from build123d import *

# Parameters (mm, degrees)
F1_DEPTH = 2057.4
F2_W     = 1651
F2_H     = 558.8
F3_DEPTH = 152.4
F4_R     = 101.6


with BuildPart() as f1:
    # F0 (on Right) → F1 (new body)
    with BuildSketch(Plane.YZ):
        Polygon((0, 939.8), (0, 0), (889, 0), (889, 558.8), (330.2, 558.8), (330.2, 939.8), align=None)
    extrude(amount=-F1_DEPTH)

    # F2 (on face) → F3 (cut)
    with BuildSketch(Plane.XY.offset(558.8)):
        with Locations((-1028.7, 609.6)):
            Rectangle(F2_W, F2_H)
    extrude(amount=-F3_DEPTH, mode=Mode.SUBTRACT)

    # F4
    f4_edges = [f1.edges().sort_by_distance(p)[0] for p in [
        (-1028.7, 889, 406.4),
        (-1028.7, 330.2, 939.8),
        (-203.2, 609.6, 558.8),
        (-1854.2, 609.6, 558.8),
    ]]
    fillet(f4_edges, radius=F4_R)


solid = f1.part
Source: CAD feature listing. Evaluate the final solid. Frame: model axes, mm. A direction names the side the tool comes from. Round coordinates to 2 decimals unless told otherwise and drop trailing zeros. Loops run counter-clockwise (first coordinate to the right, second up) from the corner with the lowest first, then second, coordinate; pieces in that order, holes last. Notation, with made-up numbers: M 34.25,-9 L 83.25,-9 A26 ccw 83.25,24 Z; hole C 64,33 d8. An arc over 180 degrees is marked long. Return JSON: item names as keys, results as strings. Group by question number.
1. Section query D-D on z = 667. Output: boundary loops of the cut face in (x, y), and give its area (3 significant figures).
2. Section query A-A on x = -1224.5. Output: boundary loops of the cut face in (y, z), and give its area (3 significant figures).
3. Mould query, pull axis X, two halves, no side actions, for faces 1 (the face through (-1854.2, 629, 421)), 2 (the face through (-2057.4, 339, 372)), 3 (the face through (0, 339, 372)), 4 (the face through (-172.648, 613.512, 529.828)). Classes: released by +X, released by -X, zero draft, split by the parting line, or undercut.
4. Material intervals for line 1 along X through (y, z) = (527.5, 423); line 2 along Z through (x, y) = (-869, 373.5); line 3 along Y through (x, z) = (-1134, 532), sorted ascending. Write a range as from..to.
5. Section query C-C on z = 488. Output: boundary loops of the cut face in (x, y).
6. Reachability of faces 5 (the face through (-50, 614, 558.8)), 6 (the face through (-1040, 562, 406.4)), 7 (the face through (-1014, 0, 476)) from +Z, -Z, +X, -X, +Y, -Y: full face, straight path, thin tool, end or side. Return the list, or none.
7. Pin query (flat end, axial travel): pin 1 (1 mm diameter, centred on x = -1605, z = 649, fed in from +Y); pin 2 (5 mm diameter, centred on x = -1647, y = 250, fed in from +Z). Return the tip coordinate at first contact, or that it passes through.
8. Section query B-B on y = 595.5. Output: boundary loops of the cut face in (x, z).
Checks:
{
 "1": {"outline": "M -2057.4,0 L 0,0 L 0,330.2 L -2057.4,330.2 Z", "area": "679,000 mm²"},
 "2": {"outline": "M 0,0 L 889,0 L 889,304.8 A101.6 ccw 787.4,406.4 L 330.2,406.4 L 330.2,838.2 A101.6 ccw 228.6,939.8 L 0,939.8 Z", "area": "533,000 mm²"},
 "3": {"face 1": "undercut", "face 2": "released by -X", "face 3": "released by +X", "face 4": "undercut"},
 "4": {"line 1": "x = -2057.4..-1854.2, -203.2..0", "line 2": "z = 0..406.4", "line 3": "y = 0..330.2"},
 "5": {"outline": "M -2057.4,0 L 0,0 L 0,889 L -198.42,889 L -198.42,330.2 L -1858.98,330.2 L -1858.98,889 L -2057.4,889 Z"},
 "6": {"face 5": "+Z, +X, -X, +Y", "face 6": "+Z, +Y", "face 7": "+Z, -Z, +X, -X, -Y"},
 "7": {"pin 1": "stops at y = 330.2", "pin 2": "stops at z = 938.03"},
 "8": {"outline": "M -2057.4,0 L 0,0 L 0,558.8 L -101.6,558.8 A101.6 ccw -203.2,457.2 L -203.2,406.4 L -1854.2,406.4 L -1854.2,457.2 A101.6 ccw -1955.8,558.8 L -2057.4,558.8 Z"}
}
